from build123d import *

# Parameters (mm, degrees)
F1_DEPTH = 2190
F2_T     = -2.54


# Not quite as in the source:
# - a shell that OpenCascade refuses in one call is made with other operations: the cavity is built on its own and cut out


with BuildPart() as f1:
    # F0 (on Top) → F1 (new body)
    with BuildSketch(Plane.XY):
        with BuildLine():
            Line((690, 600), (-690, 600))
            ThreePointArc((-690, 600), (-732.4264068712, 582.4264068712), (-750, 540))
            Line((-750, 540), (-750, -540))
            ThreePointArc((-750, -540), (-732.4264068712, -582.4264068712), (-690, -600))
            Line((-690, -600), (690, -600))
            ThreePointArc((690, -600), (732.4264068712, -582.4264068712), (750, -540))
            Line((750, -540), (750, 540))
            ThreePointArc((750, 540), (732.4264068712, 582.4264068712), (690, 600))
        make_face()
    extrude(amount=F1_DEPTH)

    # F2: a shell. OpenCascade refuses it in one call, so the cavity is built on its own and cut out:
    # the body offset inwards by the wall thickness, plus a prism from it out through each open face.
    f2_core = offset(f1.part, amount=F2_T, mode=Mode.PRIVATE)
    f2_exits = [f2_core.faces().sort_by_distance(p)[0] for p in [
        (0, 597.46, 1095),
    ]]
    add(f2_core, mode=Mode.SUBTRACT)
    extrude(f2_exits, amount=-F2_T, mode=Mode.SUBTRACT)


solid = f1.part
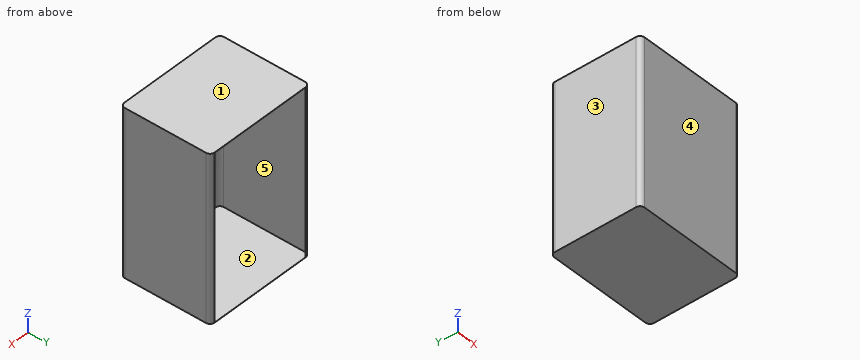
Build history of the part. All positions in model axes, mm. Face numbers are marked on the shaded views. A direction names the side the tool comes from. Round coordinates to 2 decimals unless told otherwise and drop trailing zeros. Loops run counter-clockwise (first coordinate to the right, second up) from the corner with the lowest first, then second, coordinate; pieces in that order, holes last. Notation, with made-up numbers: (82.5, -31) -> (90.5, -31) arc R21 cw to (90.5, -26) -> close; hole circle Ø11 at (61.5, 43.25). An arc over 180 degrees is marked (long way). One line per item, written item: value. Start each with the question number.
Q1. Cut at C-C on x = -387.5. List the corners of the cut face in (y, z), plus the area to 3 significant figures.
Q2. Cut at A-A on y = 28.5. List the corners of the cut face in (x, z), plus the area to 3 significant figures.
Q3. 3-axis set-ups, long thin cutter, end or side, ignore diameter. For the marked faces 4 and 5: which of +Z, -Z, +X, -X, +Y, -Y reach the whole face in a straight line?
Q4. Drop a flat-ended pin along its axis: pin 1 Ø6 at (x, z) = (281.5, 219.5) entering from +Y. Give the stop position or say it passes through.
Q5. Probe line 1 along Z through (x, y) = (-503, 382); line 2 along X through (y, z) = (535, 534); line 3 along X through (y, z) = (-547.5, 1970.5). List the from-to ranges inside material, lowest first.
Q6. Two-plate mould, pull along X, no slides. Class the marked faces 1, 2 and 3: released by +X, released by -X, zero draft, split by the parting line, or undercut.
Q7. Cut at B-B on z = 1842. List the corners of the cut face in (x, y), plus the area to 3 significant figures.
Computed:
1. outline: (-600, 0) -> (600, 0) -> (600, 2.54) -> (-597.46, 2.54) -> (-597.46, 2187.46) -> (600, 2187.46) -> (600, 2190) -> (-600, 2190) -> close
1. area: 11,600 mm²
2. outline: (-750, 0) -> (750, 0) -> (750, 2190) -> (-750, 2190) -> close; hole (-747.46, 2.54) -> (747.46, 2.54) -> (747.46, 2187.46) -> (-747.46, 2187.46) -> close
2. area: 18,700 mm²
3. face 4: +Z, -Z, +X, -X, -Y
3. face 5: none
4. pin 1: y = -597.46
5. line 1: 0 to 2.54, 2187.46 to 2190
5. line 2: -750 to -747.46, 747.46 to 750
5. line 3: -749.53 to -746.97, 746.97 to 749.53
6. face 1: zero draft
6. face 2: undercut
6. face 3: released by -X
7. outline: (-750, -540) arc R60 ccw to (-690, -600) -> (690, -600) arc R60 ccw to (750, -540) -> (750, 540) arc R60 ccw to (690, 600) -> (690, 597.46) arc R57.46 cw to (747.46, 540) -> (747.46, -540) arc R57.46 cw to (690, -597.46) -> (-690, -597.46) arc R57.46 cw to (-747.46, -540) -> (-747.46, 540) arc R57.46 cw to (-690, 597.46) -> (-690, 600) arc R60 ccw to (-750, 540) -> close
7. area: 9,930 mm²
